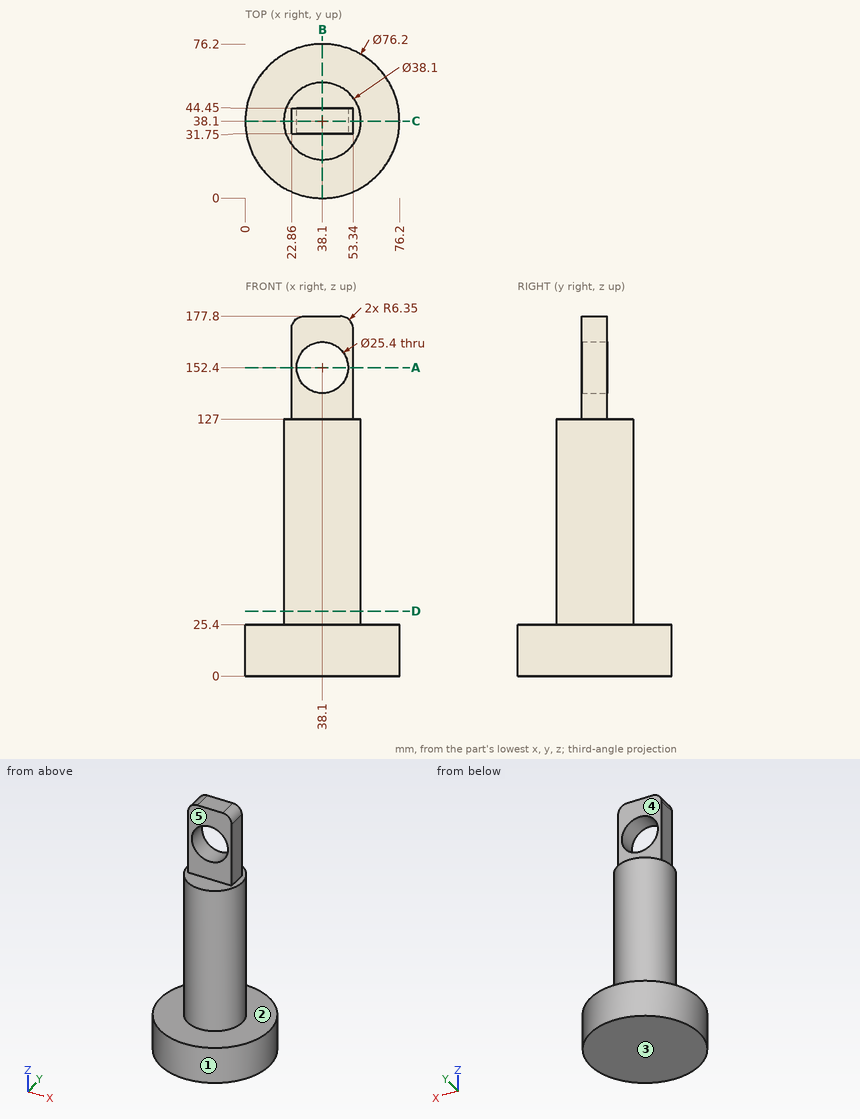
The figure shows three views and two pictorial views of one solid part (mm, origin at its lowest corner). Answer the questions. A direction names the side the tool comes from. Round coordinates to 2 decimals unless told otherwise and drop trailing zeros. Loops run counter-clockwise (first coordinate to the right, second up) from the corner with the lowest first, then second, coordinate; pieces in that order, holes last. Notation, with made-up numbers: (4.5, 69.5) -> (41.5, 69.5) arc R9 cw to (41.5, 79.5) -> close; hole circle Ø1 at (41, 67). An arc over 180 degrees is marked (long way). Use one line per item in the form item = value.
(1) Find section A-A on z = 152.4. Give the vertices of the cut face in (x, y).
Answer list:
outline = (22.86, 31.75) -> (25.4, 31.75) -> (25.4, 44.45) -> (22.86, 44.45) -> close; (50.8, 31.75) -> (53.34, 31.75) -> (53.34, 44.45) -> (50.8, 44.45) -> close
(2) Find section C-C on y = 38.1. Give the vertices of the cut face in (x, z).
Answer list:
outline = (0, 0) -> (76.2, 0) -> (76.2, 25.4) -> (57.15, 25.4) -> (57.15, 127) -> (53.34, 127) -> (53.34, 171.45) arc R6.35 ccw to (46.99, 177.8) -> (29.21, 177.8) arc R6.35 ccw to (22.86, 171.45) -> (22.86, 127) -> (19.05, 127) -> (19.05, 25.4) -> (0, 25.4) -> close; hole circle Ø25.4 at (38.1, 152.4)
(3) Flat-ended cylindrical pins translate along their axes: P1, Ø4, axis at x = 48, z = 148, coming from the -Y side; P2, Ø4, axis at x = 25, z = 29.5, coming from the -Y side; P3, Ø15, axis at x = 44, z = 165, coming from the +Y side; P4, Ø4, axis at x = 33, y = 51, coming from the -Z side. Find the tip coordinate at first contact, or state that the pin passes through.
Answer list:
P1 = 31.75
P2 = 22.62
P3 = 44.45
P4 = 0
(4) Straight lines are drawn through the part: line 1 (X direction, y = 35.75, z = 152.4); line 2 (Z direction, x = 38.1, y = 35.25); line 3 (Z direction, x = 22, y = 59.5). For each, find the intervals that lie inside material, in ascending order.
Answer list:
line_1 = 22.86 to 25.4, 50.8 to 53.34
line_2 = 0 to 139.7, 165.1 to 177.8
line_3 = 0 to 25.4
(5) Find section D-D on z = 32. Give the vertices of the cut face in (x, y), then the cut area to 3 significant figures.
Answer list:
outline = circle Ø38.1 at (38.1, 38.1)
area = 1,140 mm2
(6) Find section B-B on x = 38.1. Give the vertices of the cut face in (y, z).
Answer list:
outline = (0, 0) -> (76.2, 0) -> (76.2, 25.4) -> (57.15, 25.4) -> (57.15, 127) -> (44.45, 127) -> (44.45, 139.7) -> (31.75, 139.7) -> (31.75, 127) -> (19.05, 127) -> (19.05, 25.4) -> (0, 25.4) -> close; (31.75, 165.1) -> (44.45, 165.1) -> (44.45, 177.8) -> (31.75, 177.8) -> close
(7) A tool of negligible diameter and unlimited length cuts with its end or side. For the marked faces 1, 2, 3, 4 and 5, from which of +Z, -Z, +X, -X, +Y, -Y can it reach the whole face along a straight path? Write none if from no direction.
Answer list:
face_1 = +Z, -Z
face_2 = +Z
face_3 = -Z, +X, -X, +Y, -Y
face_4 = +Z, +X, -X, +Y
face_5 = +Z, +X, -X, -Y
